The listing builds one solid part. Answer for the finished solid, in the listing's coordinates (mm). Face numbers are marked on the shaded views. A direction names the side the tool comes from. Round coordinates to 2 decimals unless told otherwise and drop trailing zeros. Order: outer loops, then holes, each group sorted by start corner. A loop starts at its lowest first (then second) coordinate and runs counter-clockwise, first axis right, second up. Notation, with made-up numbers: M 63,-26.5 L 92,-26.5 A29 ccw 92,5.5 Z; hole C 5.25,-30.5 d5. An arc over 180 degrees is marked long. Write item = value, one per line. Start each with the question number.
(1) For a pull along Z with two mould halves and no side action, classify the marked faces 5, 6 and 7 as released by +Z, released by -Z, zero draft, split by the parting line, or undercut.
(2) A cutting plane is placed at C-C, the plane y = 2. Determine the outline of the cut face in (x, z).
(3) Which of the six approach directions +Z, -Z, +X, -X, +Y, -Y give full straight-line access (tool end or side, diameter ignored) to the marked faces 1, 2, 3 and 4?
(4) Each of these flat-tipped pins is pushed along its axis until it touches: pin 1 (0.7 mm diameter, centred on x = 0, z = 0, fed in from -Y); pin 2 (0.5 mm diameter, centred on x = 0, y = 10.5, fed in from -Z); pin 3 (3 mm diameter, centred on x = 0, z = 0, fed in from -Y); pin 4 (1 mm diameter, centred on x = -1.5, y = 4, fed in from +Z). Where does it stop, or does it pass through?
(5) Straight lines are drawn through the part: probe 1 along Z at (x, y) = (-0.1, 11.5); probe 2 along X at (y, z) = (5.75, 0); probe 3 along X at (y, z) = (8.5, 1.4). For each, find the intervals that lie inside material, in ascending order. Write a range as from..to.
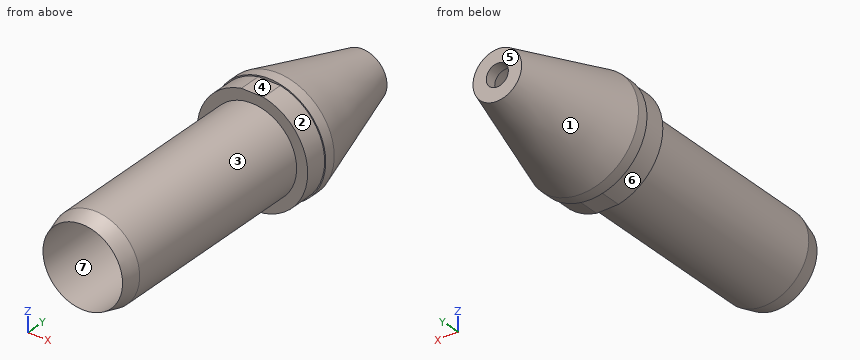
from build123d import *

# Parameters (mm, degrees)
CROQUIS2_W            = 5
CROQUIS2_H            = 0.1
CORTAR_EXTRUIR1_DEPTH = 1


with BuildPart() as part:
    # Croquis1 → Revolución1 (revolve)
    with BuildSketch(Plane.XY, mode=Mode.PRIVATE) as revoluci_n1_sk:
        Polygon((1.05, 10), (1.8, 10), (1.8, 0), (2, 0.746410162), (2, 10), (2.5, 10), (2.5, 11), (2.55, 11), (2.55, 11.5), (1.1, 16.5), (0.5, 16.5), (0.5, 16), (0.724399385, 16), (2, 11.5), (2, 10.5), (1.5, 10.5), (1.05, 10.5), align=None)
    revolve(revoluci_n1_sk.sketch.rotate(Axis((0, 0, 0), (0, 1, 0)), 90), axis=Axis((0, 0, 0), (0, 1, 0)))

    # Croquis2 → Cortar-Extruir1 (cut)
    with BuildSketch(Plane.XZ.offset(-10)):
        with Locations((0, 2.5)):
            Rectangle(CROQUIS2_W, CROQUIS2_H)
        with Locations((0, -2.5)):
            Rectangle(CROQUIS2_W, CROQUIS2_H)
    extrude(amount=-CORTAR_EXTRUIR1_DEPTH, mode=Mode.SUBTRACT)


solid = part.part
Reported:
q1.face_5 = zero draft
q1.face_6 = split by the parting line
q1.face_7 = undercut
q2.outline = C 0,0 d4; hole C 0,0 d3.6
q3.face_1 = +Y
q3.face_2 = +X, -Y
q3.face_3 = -Y
q3.face_4 = +Z, +X, -X, -Y
q4.pin_1 = through
q4.pin_2 = -2.45
q4.pin_3 = 10
q4.pin_4 = 1.73
q5.probe_1 = -2.55..-2, 2..2.55
q5.probe_2 = -2..-1.8, 1.8..2
q5.probe_3 = -1.43..-1.13, 1.13..1.43
